from build123d import *

# Parameters (mm, degrees)
SKETCH_1_R      = 0.9
EXTRUDE_1_DEPTH = 1


with BuildPart() as part:
    # Эскиз1 → Бобышка-Вытянуть1 (new body)
    with BuildSketch(Plane(origin=(0, 0, 0), x_dir=(1, 0, 0), z_dir=(0, 1, 0))):
        with BuildLine():
            Line((-2.955209453, 0.158565738), (-2.658114772, 1.301088723))
            ThreePointArc((-2.658114772, 1.301088723), (-2.611972769, 1.36215246), (-2.536166863, 1.372703719))
            Line((-2.536166863, 1.372703719), (-2.390204654, 1.3347486))
            ThreePointArc((-2.390204654, 1.3347486), (-2.157733286, 1.344214113), (-1.969855467, 1.481452804))
            ThreePointArc((-1.969855467, 1.481452804), (-1.966473238, 1.485939425), (-1.96308079, 1.490418325))
            ThreePointArc((-1.96308079, 1.490418325), (-1.882365193, 1.708632727), (-1.936743933, 1.934852721))
            Line((-1.936743933, 1.934852721), (-2.013116479, 2.064901911))
            ThreePointArc((-2.013116479, 2.064901911), (-2.023667738, 2.140707816), (-1.977525735, 2.201771553))
            Line((-1.977525735, 2.201771553), (-0.959562321, 2.799579639))
            ThreePointArc((-0.959562321, 2.799579639), (-0.883756416, 2.810130898), (-0.822692679, 2.763988896))
            Line((-0.822692679, 2.763988896), (-0.746320133, 2.633939706))
            ThreePointArc((-0.746320133, 2.633939706), (-0.575244924, 2.476250753), (-0.345352836, 2.440443482))
            ThreePointArc((-0.345352836, 2.440443482), (-0.339788718, 2.441224406), (-0.334222834, 2.441992643))
            ThreePointArc((-0.334222834, 2.441992643), (-0.122847405, 2.539218981), (-0.001337289, 2.737632248))
            Line((-0.001337289, 2.737632248), (0.03661783, 2.883594457))
            ThreePointArc((0.03661783, 2.883594457), (0.082759833, 2.944658194), (0.158565738, 2.955209453))
            Line((0.158565738, 2.955209453), (1.301088723, 2.658114772))
            ThreePointArc((1.301088723, 2.658114772), (1.36215246, 2.611972769), (1.372703719, 2.536166863))
            Line((1.372703719, 2.536166863), (1.3347486, 2.390204654))
            ThreePointArc((1.3347486, 2.390204654), (1.344214113, 2.157733286), (1.481452804, 1.969855467))
            ThreePointArc((1.481452804, 1.969855467), (1.485939425, 1.966473238), (1.490418325, 1.96308079))
            ThreePointArc((1.490418325, 1.96308079), (1.708632727, 1.882365193), (1.934852721, 1.936743933))
            Line((1.934852721, 1.936743933), (2.064901911, 2.013116479))
            ThreePointArc((2.064901911, 2.013116479), (2.140707816, 2.023667738), (2.201771553, 1.977525735))
            Line((2.201771553, 1.977525735), (2.799579639, 0.959562321))
            ThreePointArc((2.799579639, 0.959562321), (2.810130898, 0.883756416), (2.763988896, 0.822692679))
            Line((2.763988896, 0.822692679), (2.633939706, 0.746320133))
            ThreePointArc((2.633939706, 0.746320133), (2.476250753, 0.575244924), (2.440443482, 0.345352836))
            ThreePointArc((2.440443482, 0.345352836), (2.441224406, 0.339788718), (2.441992643, 0.334222834))
            ThreePointArc((2.441992643, 0.334222834), (2.539218981, 0.122847405), (2.737632248, 0.001337289))
            Line((2.737632248, 0.001337289), (2.883594457, -0.03661783))
            ThreePointArc((2.883594457, -0.03661783), (2.944658194, -0.082759833), (2.955209453, -0.158565738))
            Line((2.955209453, -0.158565738), (2.658114772, -1.301088723))
            ThreePointArc((2.658114772, -1.301088723), (2.611972769, -1.36215246), (2.536166863, -1.372703719))
            Line((2.536166863, -1.372703719), (2.390204654, -1.3347486))
            ThreePointArc((2.390204654, -1.3347486), (2.157733286, -1.344214113), (1.969855467, -1.481452804))
            ThreePointArc((1.969855467, -1.481452804), (1.966473238, -1.485939425), (1.96308079, -1.490418325))
            ThreePointArc((1.96308079, -1.490418325), (1.882365193, -1.708632727), (1.936743933, -1.934852721))
            Line((1.936743933, -1.934852721), (2.013116479, -2.064901911))
            ThreePointArc((2.013116479, -2.064901911), (2.023667738, -2.140707816), (1.977525735, -2.201771553))
            Line((1.977525735, -2.201771553), (0.959562321, -2.799579639))
            ThreePointArc((0.959562321, -2.799579639), (0.883756416, -2.810130898), (0.822692679, -2.763988896))
            Line((0.822692679, -2.763988896), (0.746320133, -2.633939706))
            ThreePointArc((0.746320133, -2.633939706), (0.575244924, -2.476250753), (0.345352836, -2.440443482))
            ThreePointArc((0.345352836, -2.440443482), (0.339788718, -2.441224406), (0.334222834, -2.441992643))
            ThreePointArc((0.334222834, -2.441992643), (0.122847405, -2.539218981), (0.001337289, -2.737632248))
            Line((0.001337289, -2.737632248), (-0.03661783, -2.883594457))
            ThreePointArc((-0.03661783, -2.883594457), (-0.082759833, -2.944658194), (-0.158565738, -2.955209453))
            Line((-0.158565738, -2.955209453), (-1.301088723, -2.658114772))
            ThreePointArc((-1.301088723, -2.658114772), (-1.36215246, -2.611972769), (-1.372703719, -2.536166863))
            Line((-1.372703719, -2.536166863), (-1.3347486, -2.390204654))
            ThreePointArc((-1.3347486, -2.390204654), (-1.344214113, -2.157733286), (-1.481452804, -1.969855467))
            ThreePointArc((-1.481452804, -1.969855467), (-1.485939425, -1.966473238), (-1.490418325, -1.96308079))
            ThreePointArc((-1.490418325, -1.96308079), (-1.708632727, -1.882365193), (-1.934852721, -1.936743933))
            Line((-1.934852721, -1.936743933), (-2.064901911, -2.013116479))
            ThreePointArc((-2.064901911, -2.013116479), (-2.140707816, -2.023667738), (-2.201771553, -1.977525735))
            Line((-2.201771553, -1.977525735), (-2.799579639, -0.959562321))
            ThreePointArc((-2.799579639, -0.959562321), (-2.810130898, -0.883756416), (-2.763988896, -0.822692679))
            Line((-2.763988896, -0.822692679), (-2.633939706, -0.746320133))
            ThreePointArc((-2.633939706, -0.746320133), (-2.476250753, -0.575244924), (-2.440443482, -0.345352836))
            ThreePointArc((-2.440443482, -0.345352836), (-2.441224406, -0.339788718), (-2.441992643, -0.334222834))
            ThreePointArc((-2.441992643, -0.334222834), (-2.539218981, -0.122847405), (-2.737632248, -0.001337289))
            Line((-2.737632248, -0.001337289), (-2.883594457, 0.03661783))
            ThreePointArc((-2.883594457, 0.03661783), (-2.944658194, 0.082759833), (-2.955209453, 0.158565738))
        make_face()
        with Locations(Location((0, 0, 0), (0, 0, 270))):
            Circle(SKETCH_1_R, mode=Mode.SUBTRACT)
    extrude(amount=EXTRUDE_1_DEPTH)


solid = part.part
Work out the finished part from the listing and answer in its coordinate system (mm). Coordinates: 2 decimals unless noted, no trailing zeros. Loops run counter-clockwise (first coordinate to the right, second up) from the corner with the lowest first, then second, coordinate; pieces in that order, holes last. Notation, with made-up numbers: (11.5, 71.25) -> (51.5, 71.25) arc R25 ccw to (51.5, 93.25) -> close; hole circle Ø8 at (46, 2). An arc over 180 degrees is marked (long way). Answer as CSV lines item,"result".
1) For a pull along Z with two mould halves and no side action, classify faces 1 (the face through (0.72, 0.49, -2.81)), 2 (the face through (-0.345, 0.493, 0.831)), 3 (the face through (-0.72, 0.49, 2.81)) as released by +Z, released by -Z, zero draft, split by the parting line, or undercut.
A:
face 1,"released by -Z"
face 2,"undercut"
face 3,"released by +Z"
2) A flat-ended cylindrical pin translates along its axis: pin 1 (1.5 mm diameter, centred on x = 1.5, z = -2.5, fed in from +Y). Find the tip coordinate at first contact, or state that the pin passes through.
A:
pin 1,"stops at y = 1"
3) Straight lines are drawn through the part: probe 1 along X at (y, z) = (0.3, 0.65); probe 2 along X at (y, z) = (0.55, 0.1); probe 3 along Z at (x, y) = (2.6, 0.2). For each, find the intervals that lie inside material, in ascending order.
A:
probe 1,"x = -2.52 to -0.62, 0.62 to 2.83"
probe 2,"x = -2.56 to -0.89, 0.89 to 2.95"
probe 3,"z = -1.3 to -0.72, -0.07 to 1.37"
4) The part is cut by section A-A (x = -0.6). Give the vertices of the cut face in (y, z).
A:
outline,"(0, -2.49) -> (1, -2.49) -> (1, -0.67) -> (0, -0.67) -> close; (0, 0.67) -> (1, 0.67) -> (1, 2.84) -> (0, 2.84) -> close"
